Verification items for this drawing (mm, ordinates from the low corner). A direction names the side the tool comes from. Give positions to 0.01 mm unless a question says otherwise; leave off trailing zeros. Write each loop counter-clockwise with the first axis right and the second up, starting at its lowest first coordinate (ties: lowest second). Pieces come first, ordered by that corner, then holes. Notation, with made-up numbers: (9.5, 30.25) -> (61.5, 30.25) arc R29 cw to (61.5, 58.25) -> close; hole circle Ø8 at (40, 27). An arc over 180 degrees is marked (long way). Answer as a JSON object with one key per item and string values.
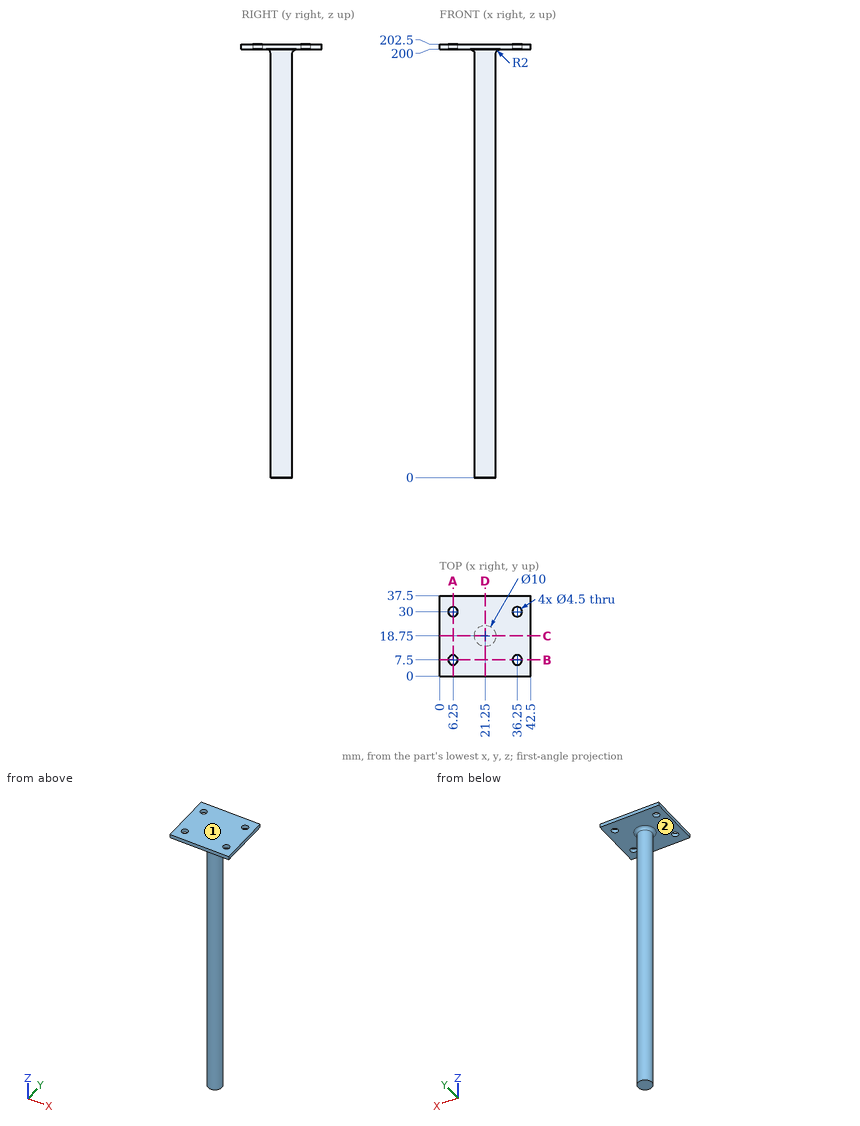
1. Sectioned sample at D-D, the plane x = 21.25. Enter the section's corners in (y, z).
Determined:
{"outline": "(0, 200) -> (11.75, 200) arc R2 cw to (13.75, 198) -> (13.75, 0) -> (23.75, 0) -> (23.75, 198) arc R2 cw to (25.75, 200) -> (37.5, 200) -> (37.5, 202.5) -> (0, 202.5) -> close"}
2. Access from +Z, -Z, +X, -X, +Y, -Y to the whole of each face (thin tool, end or side, straight path). Record for the marked faces 1 and 2.
Determined:
{"face 1": "+Z, +X, -X, +Y, -Y", "face 2": "-Z"}
3. Sectioned sample at A-A, the plane x = 6.25. Enter the section's corners in (y, z), plus the area to 4 significant figures.
Determined:
{"outline": "(0, 200) -> (5.25, 200) -> (5.25, 202.5) -> (0, 202.5) -> close; (9.75, 200) -> (27.75, 200) -> (27.75, 202.5) -> (9.75, 202.5) -> close; (32.25, 200) -> (37.5, 200) -> (37.5, 202.5) -> (32.25, 202.5) -> close", "area": "71.25 mm^2"}
4. Sectioned sample at C-C, the plane y = 18.75. Enter the section's corners in (x, z).
Determined:
{"outline": "(0, 200) -> (14.25, 200) arc R2 cw to (16.25, 198) -> (16.25, 0) -> (26.25, 0) -> (26.25, 198) arc R2 cw to (28.25, 200) -> (42.5, 200) -> (42.5, 202.5) -> (0, 202.5) -> close"}
5. Scan lines: L1, parallel to Y at x = 36.25, z = 201.05; L2, parallel to Z at x = 13.5, y = 30; L3, parallel to Y at x = 24, z = 149.5. Record each from-to range of solid material in increasing order. Write a range as [from, to].
Determined:
{"L1": "[0, 5.25], [9.75, 27.75], [32.25, 37.5]", "L2": "[200, 202.5]", "L3": "[14.57, 22.93]"}
6. Sectioned sample at B-B, the plane y = 7.5. Enter the section's corners in (x, z), plus the area to 4 significant figures.
Determined:
{"outline": "(0, 200) -> (4, 200) -> (4, 202.5) -> (0, 202.5) -> close; (8.5, 200) -> (34, 200) -> (34, 202.5) -> (8.5, 202.5) -> close; (38.5, 200) -> (42.5, 200) -> (42.5, 202.5) -> (38.5, 202.5) -> close", "area": "83.75 mm^2"}
7. Go/stop test with flat-tipped pins: P1, Ø3, axis at y = 22.5, z = 168.5, coming from the -X side; P2, Ø3, axis at x = 26, z = 63, coming from the -Y side; P3, Ø6, axis at y = 18, z = 80.5, coming from the +X side; P4, Ø4, axis at x = 36.25, y = 7.5, coming from the -Z side. Record where each tip stops, or that it passes through.
Determined:
{"P1": "x = 16.78", "P2": "y = 14.95", "P3": "x = 26.25", "P4": "through"}
